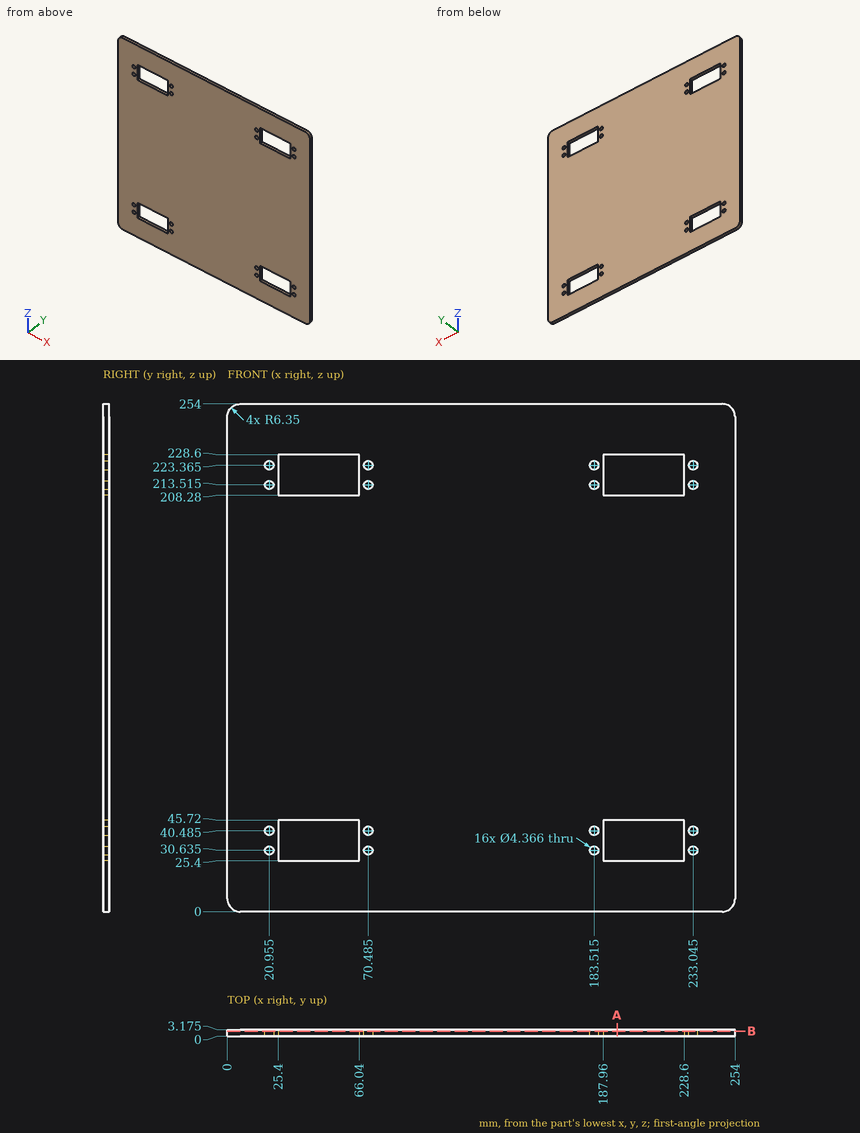
Here's the drawing with two shaded views (mm, measured from the low corner). I have some questions. Give positions to 0.01 mm unless a question says otherwise; leave off trailing zeros. Order: outer loops, then holes, each group sorted by start corner. A loop starts at its lowest first (then second) coordinate and runs counter-clockwise, first axis right, second up. Notation, with made-up numbers: (27, 54) - (84, 54) arc R19 cw to (84, 87) - close; hole circle Ø11 at (45.25, 21). An arc over 180 degrees is marked (long way). Write each question's results on one line, items separated by ' | '.
1) Please list where these lines run through material, in increasing order: line 1 along Z through (x, y) = (34, 1.75); line 2 along Z through (x, y) = (69.5, 2). Write a range as [from, to].
Final values:
line 1: z = [0, 25.4], [45.72, 208.28], [228.6, 254] | line 2: z = [0, 28.69], [32.58, 38.54], [42.43, 211.57], [215.46, 221.42], [225.31, 254]
2) I'm going to push a flat-ended pin straight in: pin 1 Ø3.5 at (x, z) = (233.045, 213.515) entering from +Y. Where does the tip first touch, or does it pass through?
Final values:
pin 1: passes through
3) Suppose I cut it at A-A, the plane x = 195. Write out the boundary of the cut face in (y, z) (1 decimal).
Final values:
outline: (0, 0) - (3.2, 0) - (3.2, 25.4) - (0, 25.4) - close; (0, 45.7) - (3.2, 45.7) - (3.2, 208.3) - (0, 208.3) - close; (0, 228.6) - (3.2, 228.6) - (3.2, 254) - (0, 254) - close
4) Suppose I cut it at B-B, the plane y = 2.5. Give the number of separate pieces and of enclosed holes in the cut face, then the cut area to 3 significant figures.
Final values:
separate pieces: 1 | enclosed holes: 20 | area: 60,900 mm^2
